Autodesk Inventor part; units mm, degrees
ref_plane "YZ Plane" through (0, 0, 0) normal (1, 0, 0) x (0, 1, 0)
ref_plane "XZ Plane" through (0, 0, 0) normal (0, 1, 0) x (-1, 0, 0)
ref_plane "XY Plane" through (0, 0, 0) normal (0, 0, 1) x (1, 0, 0)
sketch "Sketch1" plane through (0, 0, 0) normal (0, 1, 0) x (-1, 0, 0)
  circle A0 centre (0, 0) radius 4
  arc A1 (-5.8378, -12.1725) -> (-5.8378, 12.1725) centre (0, 0) ccw
  circle A2 centre (18.5, 0) radius 2.5
  circle A3 centre (-18.5, 0) radius 2.5
  line L0 (0, -18.9) -> (0, 18.9)
  line L1 (20.8784, 4.9592) -> (5.8378, 12.1725)
  line L2 (33.6, 0) -> (-33.6, 0)
  line L3 (20.8784, -4.9592) -> (5.8378, -12.1725)
  line L4 (-20.8784, 4.9592) -> (-5.8378, 12.1725)
  line L5 (-20.8784, -4.9592) -> (-5.8378, -12.1725)
  arc A4 (-20.8784, 4.9592) -> (-20.8784, -4.9592) centre (-18.5, 0) ccw
  arc A5 (20.8784, -4.9592) -> (20.8784, 4.9592) centre (18.5, 0) ccw
  dimension "d0" = 8
  dimension "d1" = 27
  dimension "d2" = 5
  dimension "d3" = 5
  dimension "d4" = 37
  dimension "d5" = 18.5
extrude "Extrusion1" add sketch "Sketch1" along normal blind 4 contours L2 A1 L0 A0 | A0 L0 A1 L2 | A0 L2 A3 A4 L4 A1 L0 | L0 A1 L5 A4 L2 A3 A0 | L2 A2 A5 L3 A1 | A1 L1 A5 L2 A2
sketch "Sketch2" plane through (0, 0, 0) normal (0, -1, 0) x (1, 0, 0)
  circle A0 centre (0, 0) radius 4
  circle A1 centre (0, 0) radius 13
  dimension "d11" = 26
extrude "Extrusion2" add sketch "Sketch2" along normal blind 4.5
sketch "Sketch3" plane through (0, -4.5, 0) normal (0, -1, 0) x (1, 0, 0)
  circle A0 centre (0, 0) radius 4
  circle A1 centre (0, 0) radius 4
  circle A2 centre (0, 0) radius 5.5
  dimension "d14" = 11
extrude "Extrusion3" add sketch "Sketch3" along normal blind 3.5
sketch "Sketch4" plane through (0, -4.5, 0) normal (0, -1, 0) x (1, 0, 0)
  circle A0 centre (0, 0) radius 5.5
  circle A1 centre (0, 0) radius 5.5
  circle A2 centre (0, 0) radius 11
  dimension "d17" = 22
extrude "Extrusion4" cut sketch "Sketch4" against normal blind 0.5
sketch "Sketch5" plane through (0, -4, 0) normal (0, -1, 0) x (1, 0, 0)
  circle A0 centre (0, 0) radius 5.5
  circle A1 centre (0, 0) radius 10.5
  dimension "d20" = 21
extrude "Extrusion5" cut sketch "Sketch5" against normal blind 0.2
properties part number "Kep Truc KLF-08"
Here's how the part is built. I have some questions about the finished solid (model axes, mm). A direction names the side the tool comes from. Give positions to 0.01 mm unless a question says otherwise; leave off trailing zeros. Loops run counter-clockwise (first coordinate to the right, second up) from the corner with the lowest first, then second, coordinate; pieces in that order, holes last. Notation, with made-up numbers: M 26.25,-29.75 L 48.25,-29.75 A21 ccw 48.25,-4.75 Z; hole C 34.25,29 d2. An arc over 180 degrees is marked long. Use one line per item in the form item = value. Start each with the question number.
Q1. Will these pins go through, and if not, where does the flat tip stop? pin 1 Ø13.5 at (x, z) = (-3, 5.5) entering from -Y; pin 2 Ø8 at (x, z) = (-18.5, 0) entering from -Y; pin 3 Ø1 at (x, y) = (16.5, 0) entering from +Z; pin 4 Ø8 at (x, z) = (-7, -7.5) entering from -Y.
Q2. I need wall thicknesses on line 1 along X through (y, z) = (1.15, 0); line 2 along Z through (x, y) = (0, -3.9); line 3 along Z through (x, y) = (0, 2.2). Which ranges of each line are inside material? Lowest first, please.
Q3. If we section it at D-D (z = 7.75): Write out the boundary of the cut face in (x, y).
Q4. If we section it at A-A (y = 3.25): Write out the boundary of the cut face in (x, z), then the cut area to 3 significant figures.
Q5. Thinking about a two-plate mould opening in Z: for faces 3 (the cylindrical face through (-16, 2, 0)), 4 (the cylindrical face through (-0.1, 2, -13.5)), 5 (the flat face through (-5, 4, 0)), which applies, +Z half, -Z half, draft (parallel to the pull), parting line (faces both ways), or undercut?
Q6. If we section it at C-C (z = 0): State how many separate pieces and enclosed holes the cut face has, then the cut area to 3 significant figures.
Q7. If we section it at B-B (x = 0): Write out the boundary of the cut face in (y, z), then the cut area to 3 significant figures.
Q8. Which directions (+Z, -Z, +X, -X, +Y, -Y) give clear straight access to the entire face, cutting with the end or side of a thin tool? Please do faces 1 (the cylindrical face through (24, 2, 0)), 2 (the cylindrical face through (-2.38, -4.25, -10.74)).
Taken from the geometry:
q1.pin_1 = -8
q1.pin_2 = 0
q1.pin_3 = 7.3
q1.pin_4 = -4.5
q2.line_1 = -24 to -21, -16 to -4, 4 to 16, 21 to 24
q2.line_2 = -13 to -10.5, -5.5 to -4, 4 to 5.5, 10.5 to 13
q2.line_3 = -13.5 to -4, 4 to 13.5
q3.outline = M -15.06,0 L -10.44,0 L -10.44,-4.5 L -7.81,-4.5 L -7.81,-4 L -7.08,-4 L -7.08,-3.8 L 7.08,-3.8 L 7.08,-4 L 7.81,-4 L 7.81,-4.5 L 10.44,-4.5 L 10.44,0 L 15.06,0 L 15.06,4 L -15.06,4 Z
q4.outline = M -20.88,-4.96 L -5.84,-12.17 A13.5 ccw 5.84,-12.17 L 20.88,-4.96 A5.5 ccw 20.88,4.96 L 5.84,12.17 A13.5 ccw -5.84,12.17 L -20.88,4.96 A5.5 ccw Z; hole C -18.5,0 d5; hole C 0,0 d8; hole C 18.5,0 d5
q4.area = 775 mm^2
q5.face_3 = undercut
q5.face_4 = -Z half
q5.face_5 = draft
q6.separate_pieces = 4
q6.enclosed_holes = 0
q6.area = 204 mm^2
q7.outline = M -8,-5.5 L -3.8,-5.5 L -3.8,-10.5 L -4,-10.5 L -4,-11 L -4.5,-11 L -4.5,-13 L 0,-13 L 0,-13.5 L 4,-13.5 L 4,-4 L -8,-4 Z; M -8,4 L 4,4 L 4,13.5 L 0,13.5 L 0,13 L -4.5,13 L -4.5,11 L -4,11 L -4,10.5 L -3.8,10.5 L -3.8,5.5 L -8,5.5 Z
q7.area = 160 mm^2
q8.face_1 = +X, +Y, -Y
q8.face_2 = -Y
